For this review, take the finished solid that the model builds, in its own axes (mm). A direction names the side the tool comes from. Coordinates: 2 decimals unless noted, no trailing zeros. Order: outer loops, then holes, each group sorted by start corner. A loop starts at its lowest first (then second) coordinate and runs counter-clockwise, first axis right, second up.
from build123d import *
from build123d.topology import SkipClean

# Parameters (mm, degrees)
SZKIC1_R                                           = 11.5
SZKIC1_R_2                                         = 4
DODANIE_WYCI_GNI_CIE1_DEPTH                        = 20
SZKIC3_W                                           = 11.5
SZKIC3_H                                           = 20
WYTNIJ_WYCI_GNI_CIE1_DEPTH                         = 1.5
WYTNIJ_WYCI_GNI_CIE2_DEPTH                         = 32
POG_BIENIE_STO_KOWE_POD_M3_WKR_T_Z_BEM_D           = 3.6
POG_BIENIE_STO_KOWE_POD_M3_WKR_T_Z_BEM_CSINK_D     = 6.3
POG_BIENIE_STO_KOWE_POD_M3_WKR_T_Z_BEM_CSINK_ANGLE = 90
SZKIC7_R                                           = 3.5
WYTNIJ_WYCI_GNI_CIE3_DEPTH                         = 32
SZKIC8_R                                           = 2
WYTNIJ_WYCI_GNI_CIE4_DEPTH                         = 7
DODANIE_WYCI_GNI_CIE2_START                        = 0.2
DODANIE_WYCI_GNI_CIE2_DEPTH                        = 0.2
DODANIE_WYCI_GNI_CIE3_START                        = 1.5
SZKIC10_R                                          = 11.5
DODANIE_WYCI_GNI_CIE3_DEPTH                        = 1.5
DODANIE_WYCI_GNI_CIE4_START                        = 5
SZKIC11_R                                          = 11.5
SZKIC11_W                                          = 10
SZKIC11_H                                          = 10
DODANIE_WYCI_GNI_CIE4_DEPTH                        = 5
SFAZOWANIE1_SIZE                                   = 3


with BuildPart() as part:
    # Szkic1 → Dodanie-wyciągnięcie1 (new body)
    with BuildSketch(Plane.XY):
        with Locations(Location((0, 0, 0), (0, 0, 180))):
            Circle(SZKIC1_R)
        with Locations(Location((0, 0, 0), (0, 0, 180))):
            Circle(SZKIC1_R_2, mode=Mode.SUBTRACT)
    extrude(amount=DODANIE_WYCI_GNI_CIE1_DEPTH)

    # Szkic3 → Wytnij-wyciągnięcie1 (cut)
    with BuildSketch(Plane(origin=(0, 0, 0), x_dir=(1, 0, 0), z_dir=(0, 1, 0))):
        with Locations((5.75, -10)):
            Rectangle(SZKIC3_W, SZKIC3_H)
    extrude(amount=WYTNIJ_WYCI_GNI_CIE1_DEPTH, mode=Mode.SUBTRACT)

    # Szkic4 → Wytnij-wyciągnięcie2 (cut)
    with BuildSketch(Plane(origin=(0, 4, 0), x_dir=(1, 0, 0), z_dir=(0, 1, 0))):
        with BuildLine():
            ThreePointArc((7, -11.75), (3.75, -15), (7, -18.25))
            Line((7, -18.25), (7, -11.75))
        make_face()
        with BuildLine():
            Line((7, -11.75), (7, -18.25))
            ThreePointArc((7, -18.25), (9.298097039, -17.298097039), (10.25, -15))
            ThreePointArc((10.25, -15), (9.298097039, -12.701902961), (7, -11.75))
        make_face()
        with BuildLine():
            ThreePointArc((7, -1.75), (3.75, -5), (7, -8.25))
            Line((7, -8.25), (7, -1.75))
        make_face()
        with BuildLine():
            Line((7, -1.75), (7, -8.25))
            ThreePointArc((7, -8.25), (9.298097039, -7.298097039), (10.25, -5))
            ThreePointArc((10.25, -5), (9.298097039, -2.701902961), (7, -1.75))
        make_face()
    extrude(amount=WYTNIJ_WYCI_GNI_CIE2_DEPTH, mode=Mode.SUBTRACT)

    # Pogłębienie stożkowe pod M3 Wkręt z łbem płaskim1 (through all)
    with Locations(Plane(origin=(7, 4, 15), x_dir=(0, 0, 1), z_dir=(0, 1, 0))):
        with Locations((0, 0), (-10, 0)):
            CounterSinkHole(POG_BIENIE_STO_KOWE_POD_M3_WKR_T_Z_BEM_D / 2, POG_BIENIE_STO_KOWE_POD_M3_WKR_T_Z_BEM_CSINK_D / 2, counter_sink_angle=POG_BIENIE_STO_KOWE_POD_M3_WKR_T_Z_BEM_CSINK_ANGLE)

    # Szkic7 → Wytnij-wyciągnięcie3 (cut)
    with BuildSketch(Plane(origin=(0, -6.5, 0), x_dir=(-1, 0, 0), z_dir=(0, -1, 0))):
        with Locations((-7, -5)):
            Circle(SZKIC7_R)
        with Locations((-7, -15)):
            Circle(SZKIC7_R)
    extrude(amount=WYTNIJ_WYCI_GNI_CIE3_DEPTH, mode=Mode.SUBTRACT)

    # Szkic8 → Wytnij-wyciągnięcie4 (cut)
    with BuildSketch(Plane.XZ.offset(6.5)):
        with Locations((7, 15)):
            Circle(SZKIC8_R)
        with Locations(Location((7, 5, 0), (0, 0, 90))):
            Circle(SZKIC8_R)
    extrude(amount=-WYTNIJ_WYCI_GNI_CIE4_DEPTH, mode=Mode.SUBTRACT)

    # Szkic9 → Dodanie-wyciągnięcie2 (add)
    with SkipClean():  # the faces are left unmerged after this step: merging them gives an invalid solid
        with BuildSketch(Plane(origin=(0, 0, 0), x_dir=(-1, 0, 0), z_dir=(0, 0, -1)).offset(DODANIE_WYCI_GNI_CIE2_START)):
            with BuildLine():
                Line((0, 11.5), (0, 4))
                ThreePointArc((0, 4), (4, 0), (0, -4))
                Line((0, -4), (0, -11.5))
                ThreePointArc((0, -11.5), (11.5, 0), (0, 11.5))
            make_face()
        extrude(amount=-DODANIE_WYCI_GNI_CIE2_DEPTH)

    # Szkic10 → Dodanie-wyciągnięcie3 (add)
    with SkipClean():  # the faces are left unmerged after this step: merging them gives an invalid solid
        with BuildSketch(Plane(origin=(0, 0, -0.2), x_dir=(-1, 0, 0), z_dir=(0, 0, -1)).offset(DODANIE_WYCI_GNI_CIE3_START)):
            Circle(SZKIC10_R)
        extrude(amount=-DODANIE_WYCI_GNI_CIE3_DEPTH)

    # Szkic11 → Dodanie-wyciągnięcie4 (add)
    with SkipClean():  # the faces are left unmerged after this step: merging them gives an invalid solid
        with BuildSketch(Plane(origin=(0, 0, -1.7), x_dir=(-1, 0, 0), z_dir=(0, 0, -1)).offset(DODANIE_WYCI_GNI_CIE4_START)):
            Circle(SZKIC11_R)
            Rectangle(SZKIC11_W, SZKIC11_H, mode=Mode.SUBTRACT)
        extrude(amount=-DODANIE_WYCI_GNI_CIE4_DEPTH)

    # Sfazowanie1
    # the kernel refuses this chamfer: 3 mm, written as the material it takes off along each edge
    with BuildSketch(Plane(origin=(0, 0, 20), x_dir=(-1, 0, 0), z_dir=(0, 1, 0))) as sfazowanie1_piece_1:
        Polygon((11.5, -SFAZOWANIE1_SIZE), (11.5 - SFAZOWANIE1_SIZE, 0), (11.5, 0), align=None)
    revolve(axis=Axis((0, 0, 20), (0, 0, 1)), revolution_arc=218.500054596, mode=Mode.SUBTRACT)
    with BuildSketch(Plane(origin=(0, 0, 20), x_dir=(0.8571646812696857, -0.5150424343525863, 0), z_dir=(-0.5150424343525863, -0.8571646812696857, 0))) as sfazowanie1_piece_2:
        Polygon((11.5, -SFAZOWANIE1_SIZE), (11.5 - SFAZOWANIE1_SIZE, 0), (11.5, 0), align=None)
    revolve(axis=Axis((0, 0, 20), (0, 0, 1)), revolution_arc=211.000291399, mode=Mode.SUBTRACT)


solid = part.part
1. Take a section at C-C, the plane z = 9.75. Give the boundary of the cut face in (x, y).
Answer below:
outline: (3.71, 1.5) - (11.4, 1.5) arc R11.5 ccw (long way) to (11.5, 0) - (4, 0) arc R4 cw (long way) to start
2. Machinability: for faces 3 (the face through (8, 1.5, 10)), 4 (the face through (6, -6, 0)), 5 (the face through (3.5, -8.2, 5.1)), 6 (the face through (5, 0, -4)), which of the approach directions +Z, -Z, +X, -X, +Y, -Y give a long, thin tool a straight path to every point of the face, cutting with its end or side? Answer none if there is none.
Answer below:
face 3: +Z, +X
face 4: +X, +Y, -Y
face 5: -Y
face 6: -Z
3. Take a section at B-B, the plane y = -1. Give the number of separate pieces and of enclosed holes in the cut face, plus the area to 3 significant figures.
Answer below:
separate pieces: 2
enclosed holes: 2
area: 370 mm2
4. To check wall thickness, follow L1, parallel to Z at x = 7, y = 1.85; L2, parallel to Z at x = 7, y = -4.5; L3, parallel to Z at x = 2, y = -1.25. State the ranges of each line that lie inside material, in increasing order.
Answer below:
L1: z = -6.7 to -0.2, 0 to 3.2, 6.8 to 13.2, 16.8 to 20
L2: z = -6.7 to -0.2, 0 to 3, 7 to 13, 17 to 20
L3: z = -1.7 to -0.2
5. The part is to be moulded in two halves that separate along X. For faces 1 (the face through (5.243, 2.067, 15.39)), 2 (the face through (5, 6, 0)), say which applies: +X half, -X half, draft (parallel to the pull), parting line (faces both ways), or undercut.
Answer below:
face 1: undercut
face 2: draft
6. Take a section at A-A, the plane z = -3.5. Give the boundary of the cut face in (x, y), plus the area to 3 significant figures.
Answer below:
outline: circle Ø23 at (0, 0); hole (-5, -5) - (5, -5) - (5, 5) - (-5, 5) - close
area: 315 mm2
7. Clearance check with flat-ended pins moving along their axes: pin 1 Ø8.5 at (x, z) = (7, 7) entering from -Y; pin 2 Ø1 at (x, z) = (-8.5, 7.5) entering from -Y; pin 3 Ø5 at (x, z) = (7, 5) entering from +Y; pin 4 Ø1.8 at (x, z) = (7, 15.5) entering from -Y. State where each tip first meets the part, or that it passes through.
Answer below:
pin 1: stops at y = -11.17
pin 2: stops at y = -8.26
pin 3: stops at y = 3.35
pin 4: passes through
